```python
from build123d import *

# Parameters (mm, degrees)
F3_DEPTH = 19.05
F4_R     = 1.27
F5_R     = 1.143
F6_DEPTH = 19.051
F5_R_2   = 1.524
F7_DEPTH = 2.54


with BuildPart() as f1:
    # F0 (on Front) → F1 (revolve)
    with BuildSketch(Plane.XZ):
        with BuildLine():
            Line((44.45, 0), (44.45, 19.05))
            Line((44.45, 19.05), (32.5831812388, 19.05))
            Line((32.5831812388, 19.05), (31.8430524831, 19.05))
            add(Edge.make_bspline(
                [(31.8430524831, 19.05), (30.8689221212, 18.9802011565), (29.8627306323, 16.2488706166), (28.0966354441, 15.4760789224), (26.3999857389, 13.3501170166), (25.1129431354, 15.4487673344), (22.290366868, 14.8911495391), (20.2790890798, 12.2640383952), (16.1024312734, 10.2245936819), (12.2327761722, 12.1993870362), (6.3942289854, 14.4550088103), (0, 14.3365386442)],
                knots=[0, 0, 0, 0, 0.1060699652, 0.1932935704, 0.2769325799, 0.3540227049, 0.4454383371, 0.554157978, 0.6746311283, 0.787205531, 1, 1, 1, 1], degree=3))
            Line((0, 14.3365386442), (0, 0))
            Line((0, 0), (44.45, 0))
        make_face()
    revolve(axis=Axis((0, 0, 7.1682693221), (0, 0, -1)))

    # F2 (on face) → F3 (join, through all)
    with BuildSketch(Plane(origin=(0, 0, 0), x_dir=(1, 0, 0), z_dir=(0, 0, -1))):
        with BuildLine():
            ThreePointArc((0, -44.45), (-31.4308964559, -31.4308963916), (-44.45, 9.1e-08))
            Line((-44.45, 9.1e-08), (-44.45, -44.45))
            Line((-44.45, -44.45), (0, -44.45))
        make_face()
        with BuildLine():
            Line((44.45, -44.45), (44.45, 0))
            ThreePointArc((44.45, 0), (31.4308964237, -31.4308964237), (0, -44.45))
            Line((0, -44.45), (44.45, -44.45))
        make_face()
        with BuildLine():
            Line((44.45, 44.45), (0, 44.45))
            ThreePointArc((0, 44.45), (31.4308964237, 31.4308964237), (44.45, 0))
            Line((44.45, 0), (44.45, 44.45))
        make_face()
        with BuildLine():
            ThreePointArc((-44.45, 9.1e-08), (-31.4308963916, 31.4308964559), (0, 44.45))
            Line((0, 44.45), (-44.45, 44.45))
            Line((-44.45, 44.45), (-44.45, 9.1e-08))
        make_face()
    extrude(amount=-F3_DEPTH)

    # F4
    f4_edges = [f1.edges().sort_by_distance(p)[0] for p in [
        (0, 44.45, 19.05),
        (44.45, 0, 19.05),
        (44.45, 44.45, 9.525),
        (44.45, -44.45, 9.525),
        (0, -44.45, 19.05),
        (-44.45, 0, 19.05),
        (-44.45, 44.45, 9.525),
        (-44.45, -44.45, 9.525),
    ]]
    fillet(f4_edges, radius=F4_R)

    # F5 (on face) → F6 (cut, through all)
    with BuildSketch(Plane.XY.offset(19.05)):
        with Locations((-33.4832191722, 33.4832191722)):
            Circle(F5_R)
        with Locations((-33.4832191722, -33.4832191722)):
            Circle(F5_R)
        with Locations((33.4832191722, -33.4832191722)):
            Circle(F5_R)
        with Locations((33.4832191722, 33.4832191722)):
            Circle(F5_R)
    extrude(amount=-F6_DEPTH, mode=Mode.SUBTRACT)

    # F5 (on face) → F7 (cut)
    with BuildSketch(Plane.XY.offset(19.05)):
        with Locations((-33.4832191722, 33.4832191722)):
            Circle(F5_R_2)
        with Locations((-33.4832191722, 33.4832191722)):
            Circle(F5_R, mode=Mode.SUBTRACT)
        with Locations((33.4832191722, 33.4832191722)):
            Circle(F5_R_2)
        with Locations((33.4832191722, 33.4832191722)):
            Circle(F5_R, mode=Mode.SUBTRACT)
        with Locations((33.4832191722, -33.4832191722)):
            Circle(F5_R_2)
        with Locations((33.4832191722, -33.4832191722)):
            Circle(F5_R, mode=Mode.SUBTRACT)
        with Locations((-33.4832191722, -33.4832191722)):
            Circle(F5_R_2)
        with Locations((-33.4832191722, -33.4832191722)):
            Circle(F5_R, mode=Mode.SUBTRACT)
    extrude(amount=-F7_DEPTH, mode=Mode.SUBTRACT)

    # F8 (on Right) → F9 (revolve, cut)
    with BuildSketch(Plane.YZ):
        Polygon((-31.75, 0), (-25.4, 0), (-19.05, 0), (-25.4, 6.35), align=None)
    revolve(axis=Axis((0, 0, 3.175), (0, 0, 1)), mode=Mode.SUBTRACT)


solid = f1.part
```
Read the model definition and answer for the solid it produces. Units are mm, in the model's axes. A direction names the side the tool comes from. Give positions to 0.01 mm unless a question says otherwise; leave off trailing zeros. One line per item, written item: value. Start each with the question number.
(1) The part is cut by section A-A (z = 12.5). State how many separate pieces and enclosed holes the cut face has, and give its area (3 significant figures).
(2) A tool of negligible diameter and unlimited length cuts with its end or side. For faces 4 (the flat face through (1, -44.45, 9)), 5 (the cylindrical face through (-32.78, -34.835, 17.798)), from which of +Z, -Z, +X, -X, +Y, -Y can it reach the whole face along a straight path? Write none if from no direction.
(3) Flat-ended cylindrical pins translate along their axes: P1, Ø1, axis at x = -22, y = -19.5, coming from the +Z side; P2, Ø3.5, axis at x = -33, y = -33.5, coming from the +Z side; P3, Ø1.8, axis at x = 33.48, y = 33.48, coming from the +Z side; P4, Ø1.5, axis at x = -33, y = 33.5, coming from the +Z side. Find the tip coordinate at first contact, or state that the pin passes through.
(4) For a pull along Y with two mould halves and no side action, classify faces 1 (the flat face through (-1, 44.45, 9)), 2 (the flat face through (-44.45, -1, 9)), 3 (the cylindrical face through (-34.625, -33.433, 8.371)) as released by +Y, released by -Y, zero draft, split by the parting line, or undercut.
(5) Straight lines are drawn through the part: L1, parallel to X at y = -33.5, z = 9; L2, parallel to X at y = -19, z = 2.75; L3, parallel to Y at x = 6.5, z = 6.25. For each, find the intervals that lie inside material, in ascending order.
Taken from the geometry:
1. separate pieces: 2
1. enclosed holes: 5
1. area: 7,010 mm^2
2. face 4: +Z, -Z, +X, -X, -Y
2. face 5: +Z
3. P1: z = 16.94
3. P2: z = 19.05
3. P3: through
3. P4: z = 16.51
4. face 1: released by +Y
4. face 2: zero draft
4. face 3: undercut
5. L1: -44.45 to -34.63, -32.34 to 32.34, 34.63 to 44.45
5. L2: -44.45 to -21.91, -10.69 to 10.69, 21.91 to 44.45
5. L3: -44.45 to -24.66, -24.45 to 24.45, 24.66 to 44.45
